Geometry: final body of the model. Coordinates: model frame, mm. A direction names the side the tool comes from. Give positions to 0.01 mm unless a question says otherwise; leave off trailing zeros. Write each loop counter-clockwise with the first axis right and the second up, starting at its lowest first coordinate (ties: lowest second). Pieces come first, ordered by that corner, then holes. Notation, with made-up numbers: (85.5, 85) -> (116.5, 85) arc R16 ccw to (116.5, 116) -> close; hole circle Ø9 at (66.5, 23). An arc over 180 degrees is marked (long way). Answer in a Markdown table with one row per item. Add a question column.
Item 1: First-contact query: P1, Ø4.5, axis at x = 12, z = -59.5, coming from the +Y side; P2, Ø2.5, axis at x = 48.94, z = -22.93, coming from the -Y side; P3, Ø4.5, axis at x = 12.065, z = -95.25, coming from the +Y side. Flat tips, straight axial feed; report the tip coordinate or a pass-through.
Item 2: Section query A-A on z = -53. Output: boundary loops of the cut face in (x, y) (3 decimals), plus the area to 3 significant figures.
Item 3: Material intervals for probe 1 along Z at (x, y) = (110, 11); probe 2 along Z at (x, y) = (61.5, 7); probe 3 along Z at (x, y) = (110.49, 6), sorted ascending. Write a range as from..to.
Item 4: Access query for faces 1 (the cylindrical face through (13.91, 5.01, -43.68)), 2 (the flat face through (108.06, 13.38, -10.78)), 3 (the flat face through (88.579, 3.131, -83.466)). Directions: +Z, -Z, +X, -X, +Y, -Y. A direction counts if a zero-diameter tool reaches every point of the face in a straight line with its end or side. Return the directions, or none.
Item 5: Section query C-C on y = 1.5. State how many separate pieces and enclosed holes the cut face has, plus the area to 3 significant figures.
Item 6: Section query B-B on x = 81.5. Output: boundary loops of the cut face in (y, z), plus the area to 3 significant figures.
Item 7: Draft query along X for faces 4 (the cylindrical face through (121.831, 8.371, -103.884)), 5 (the flat face through (86, 3, -19.765)). Return one class per face: +X half, -X half, draft (parallel to the pull), parting line (faces both ways), or undercut.
```python
from build123d import *

# Parameters (mm, degrees)
SKETCH2_W               = 122.555
SKETCH2_H               = 104.648
SKETCH2_R               = 2
SKETCH2_W_2             = 74.295
SKETCH2_H_2             = 69.53
BOSS_EXTRUDE5_DEPTH     = 16.51
SKETCH2_4_W             = 74.295
SKETCH2_4_H             = 10
SKETCH2_4_R             = 2
BOSS_EXTRUDE7_DEPTH     = 10.16
CUT_EXTRUDE1_START      = -16.51
SKETCH3_R               = 2
CUT_EXTRUDE1_DEPTH      = 6.35
FILLET1_R               = 2.54
CUT_EXTRUDE2_START      = -10.16
SKETCH4_R               = 2
CUT_EXTRUDE2_DEPTH      = 6.35
SKETCH5_R               = 2
CUT_EXTRUDE3_DEPTH      = 6.35
SKETCH6_R               = 2
CUT_EXTRUDE4_DEPTH      = 6.35
SKETCH7_R               = 2.254
SKETCH7_R_2             = 2
SUPPORTS_3D_PRINT_DEPTH = 6.35


with BuildPart() as part:
    # Sketch2 → Boss-Extrude5 (new body)
    with BuildSketch(Plane(origin=(0, 0, 0), x_dir=(1, 0, 0), z_dir=(0, 1, 0))):
        with Locations((61.2775, 52.324)):
            Rectangle(SKETCH2_W, SKETCH2_H)
        with Locations((12.065, 95.25)):
            Circle(SKETCH2_R, mode=Mode.SUBTRACT)
        with Locations((12.065, 60.198)):
            Circle(SKETCH2_R, mode=Mode.SUBTRACT)
        with Locations((12.065, 44.45)):
            Circle(SKETCH2_R, mode=Mode.SUBTRACT)
        with Locations((12.065, 9.398)):
            Circle(SKETCH2_R, mode=Mode.SUBTRACT)
        with Locations((110.49, 9.398)):
            Circle(SKETCH2_R, mode=Mode.SUBTRACT)
        with Locations((110.49, 44.45)):
            Circle(SKETCH2_R, mode=Mode.SUBTRACT)
        with Locations((110.49, 60.198)):
            Circle(SKETCH2_R, mode=Mode.SUBTRACT)
        with Locations((110.49, 95.25)):
            Circle(SKETCH2_R, mode=Mode.SUBTRACT)
        with Locations((73.744666667, 5.08)):
            Circle(SKETCH2_R, mode=Mode.SUBTRACT)
        with Locations((48.839129454, 5.150105129)):
            Circle(SKETCH2_R, mode=Mode.SUBTRACT)
        with Locations((61.2775, 52.324)):
            Rectangle(SKETCH2_W_2, SKETCH2_H_2, mode=Mode.SUBTRACT)
    extrude(amount=BOSS_EXTRUDE5_DEPTH)

    # Sketch2<4> → Boss-Extrude7 (add)
    with BuildSketch(Plane(origin=(0, 0, 0), x_dir=(1, 0, 0), z_dir=(0, 1, 0))):
        with Locations((61.2775, 22.559)):
            Rectangle(SKETCH2_4_W, SKETCH2_4_H)
        with Locations((36.533666667, 22.559)):
            Circle(SKETCH2_4_R, mode=Mode.SUBTRACT)
        with Locations((48.939224409, 22.929823378)):
            Circle(SKETCH2_4_R, mode=Mode.SUBTRACT)
        with Locations((61.341, 22.559)):
            Circle(SKETCH2_4_R, mode=Mode.SUBTRACT)
        with Locations((73.744666667, 22.86)):
            Circle(SKETCH2_4_R, mode=Mode.SUBTRACT)
        with Locations((86.148333333, 22.559)):
            Circle(SKETCH2_4_R, mode=Mode.SUBTRACT)
        with Locations((61.2775, 82.089)):
            Rectangle(SKETCH2_4_W, SKETCH2_4_H)
        with Locations((36.533666667, 82.089)):
            Circle(SKETCH2_4_R, mode=Mode.SUBTRACT)
        with Locations((61.341, 82.089)):
            Circle(SKETCH2_4_R, mode=Mode.SUBTRACT)
        with Locations((86.148333333, 82.089)):
            Circle(SKETCH2_4_R, mode=Mode.SUBTRACT)
    extrude(amount=BOSS_EXTRUDE7_DEPTH)

    # Sketch3 → Cut-Extrude1 (cut)
    with BuildSketch(Plane.XZ.offset(CUT_EXTRUDE1_START)):
        Polygon((13.678116652, -6.604), (10.451883348, -6.604), (8.838766696, -9.398), (10.451883348, -12.192), (13.678116652, -12.192), (15.291233304, -9.398), align=None)
        with Locations((12.065, -9.398)):
            Circle(SKETCH3_R, mode=Mode.SUBTRACT)
        Polygon((13.678116652, -92.456), (10.451883348, -92.456), (8.838766696, -95.25), (10.451883348, -98.044), (13.678116652, -98.044), (15.291233304, -95.25), align=None)
        with Locations((12.065, -95.25)):
            Circle(SKETCH3_R, mode=Mode.SUBTRACT)
        Polygon((112.103116652, -92.456), (108.876883348, -92.456), (107.263766696, -95.25), (108.876883348, -98.044), (112.103116652, -98.044), (113.716233304, -95.25), align=None)
        with Locations((110.49, -95.25)):
            Circle(SKETCH3_R, mode=Mode.SUBTRACT)
        Polygon((108.876883348, -12.192), (112.103116652, -12.192), (113.716233304, -9.398), (112.103116652, -6.604), (108.876883348, -6.604), (107.263766696, -9.398), align=None)
        with Locations((110.49, -9.398)):
            Circle(SKETCH3_R, mode=Mode.SUBTRACT)
        Polygon((13.678116652, -62.992), (15.291233304, -60.198), (13.678116652, -57.404), (10.451883348, -57.404), (8.838766696, -60.198), (10.451883348, -62.992), align=None)
        with Locations((12.065, -60.198)):
            Circle(SKETCH3_R, mode=Mode.SUBTRACT)
        Polygon((8.838766696, -44.45), (10.451883348, -47.244), (13.678116652, -47.244), (15.291233304, -44.45), (13.678116652, -41.656), (10.451883348, -41.656), align=None)
        with Locations((12.065, -44.45)):
            Circle(SKETCH3_R, mode=Mode.SUBTRACT)
        Polygon((107.263766696, -44.45), (108.876883348, -47.244), (112.103116652, -47.244), (113.716233304, -44.45), (112.103116652, -41.656), (108.876883348, -41.656), align=None)
        with Locations((110.49, -44.45)):
            Circle(SKETCH3_R, mode=Mode.SUBTRACT)
        Polygon((108.876883348, -57.404), (107.263766696, -60.198), (108.876883348, -62.992), (112.103116652, -62.992), (113.716233304, -60.198), (112.103116652, -57.404), align=None)
        with Locations((110.49, -60.198)):
            Circle(SKETCH3_R, mode=Mode.SUBTRACT)
    extrude(amount=CUT_EXTRUDE1_DEPTH, mode=Mode.SUBTRACT)

    # Fillet1
    fillet1_edges = [part.edges().sort_by_distance(p)[0] for p in [
        (0, 8.255, 0),
        (0, 8.255, -104.648),
        (122.555, 8.255, -104.648),
        (122.555, 8.255, 0),
    ]]
    fillet(fillet1_edges, radius=FILLET1_R)

    # Sketch4 → Cut-Extrude2 (cut)
    with BuildSketch(Plane(origin=(0, 10.16, 0), x_dir=(1, 0, 0), z_dir=(0, 1, 0)).offset(CUT_EXTRUDE2_START)):
        Polygon((39.759899971, 22.559), (38.146783319, 25.353), (34.920550015, 25.353), (33.307433362, 22.559), (34.920550015, 19.765), (38.146783319, 19.765), align=None)
        with Locations((36.533666667, 22.559)):
            Circle(SKETCH4_R, mode=Mode.SUBTRACT)
        Polygon((58.114766696, 22.559), (59.727883348, 19.765), (62.954116652, 19.765), (64.567233304, 22.559), (62.954116652, 25.353), (59.727883348, 25.353), align=None)
        with Locations((61.341, 22.559)):
            Circle(SKETCH4_R, mode=Mode.SUBTRACT)
        Polygon((82.922100029, 22.559), (84.535216681, 19.765), (87.761449985, 19.765), (89.374566638, 22.559), (87.761449985, 25.353), (84.535216681, 25.353), align=None)
        with Locations((86.148333333, 22.559)):
            Circle(SKETCH4_R, mode=Mode.SUBTRACT)
        Polygon((82.922100029, 82.089), (84.535216681, 79.295), (87.761449985, 79.295), (89.374566638, 82.089), (87.761449985, 84.883), (84.535216681, 84.883), align=None)
        with Locations((86.148333333, 82.089)):
            Circle(SKETCH4_R, mode=Mode.SUBTRACT)
        Polygon((64.567233304, 82.089), (62.954116652, 84.883), (59.727883348, 84.883), (58.114766696, 82.089), (59.727883348, 79.295), (62.954116652, 79.295), align=None)
        with Locations((61.341, 82.089)):
            Circle(SKETCH4_R, mode=Mode.SUBTRACT)
        Polygon((39.759899971, 82.089), (38.146783319, 84.883), (34.920550015, 84.883), (33.307433362, 82.089), (34.920550015, 79.295), (38.146783319, 79.295), align=None)
        with Locations((36.533666667, 82.089)):
            Circle(SKETCH4_R, mode=Mode.SUBTRACT)
    extrude(amount=CUT_EXTRUDE2_DEPTH, mode=Mode.SUBTRACT)

    # Sketch5 → Cut-Extrude3 (cut)
    with BuildSketch(Plane(origin=(0, 10.16, 0), x_dir=(1, 0, 0), z_dir=(0, 1, 0))):
        with Locations((48.839129454, 5.150105129)):
            Circle(SKETCH5_R)
        with Locations((73.744666667, 5.08)):
            Circle(SKETCH5_R)
        Polygon((76.970899971, 22.86), (75.357783319, 25.654), (72.131550015, 25.654), (70.518433362, 22.86), (72.131550015, 20.066), (75.357783319, 20.066), align=None)
        with Locations((73.744666667, 22.86)):
            Circle(SKETCH5_R, mode=Mode.SUBTRACT)
        Polygon((52.165457714, 22.929823378), (50.552341061, 25.723823378), (47.326107757, 25.723823378), (45.712991105, 22.929823378), (47.326107757, 20.135823378), (50.552341061, 20.135823378), align=None)
        with Locations((48.939224409, 22.929823378)):
            Circle(SKETCH5_R, mode=Mode.SUBTRACT)
    extrude(amount=-CUT_EXTRUDE3_DEPTH, mode=Mode.SUBTRACT)

    # Sketch6 → Cut-Extrude4 (cut)
    with BuildSketch(Plane(origin=(0, 16.51, 0), x_dir=(1, 0, 0), z_dir=(0, 1, 0))):
        Polygon((70.518433362, 5.08), (72.131550015, 2.286), (75.357783319, 2.286), (76.970899971, 5.08), (75.357783319, 7.874), (72.131550015, 7.874), align=None)
        with Locations((73.744666667, 5.08)):
            Circle(SKETCH6_R, mode=Mode.SUBTRACT)
        Polygon((45.612896149, 5.150105129), (47.226012801, 2.356105129), (50.452246106, 2.356105129), (52.065362758, 5.150105129), (50.452246106, 7.944105129), (47.226012801, 7.944105129), align=None)
        with Locations((48.839129454, 5.150105129)):
            Circle(SKETCH6_R, mode=Mode.SUBTRACT)
    extrude(amount=-CUT_EXTRUDE4_DEPTH, mode=Mode.SUBTRACT)

    # Sketch7 → Supports - 3D Print (add)
    with BuildSketch(Plane.XZ.offset(-6.35)):
        with Locations((36.533666667, -82.089)):
            Circle(SKETCH7_R)
        with Locations((36.533666667, -82.089)):
            Circle(SKETCH7_R_2, mode=Mode.SUBTRACT)
        with Locations((61.341, -82.089)):
            Circle(SKETCH7_R)
        with Locations((61.341, -82.089)):
            Circle(SKETCH7_R_2, mode=Mode.SUBTRACT)
        with Locations((86.148333333, -82.089)):
            Circle(SKETCH7_R)
        with Locations((86.148333333, -82.089)):
            Circle(SKETCH7_R_2, mode=Mode.SUBTRACT)
        with Locations((86.148333333, -22.559)):
            Circle(SKETCH7_R)
        with Locations((86.148333333, -22.559)):
            Circle(SKETCH7_R_2, mode=Mode.SUBTRACT)
        with Locations((61.341, -22.559)):
            Circle(SKETCH7_R)
        with Locations((61.341, -22.559)):
            Circle(SKETCH7_R_2, mode=Mode.SUBTRACT)
        with Locations((36.533666667, -22.559)):
            Circle(SKETCH7_R)
        with Locations((36.533666667, -22.559)):
            Circle(SKETCH7_R_2, mode=Mode.SUBTRACT)
    extrude(amount=SUPPORTS_3D_PRINT_DEPTH)


solid = part.part
```
Findings below:
| question | item | result |
|---|---|---|
| 1 | P1 | stops at y = 16.51 |
| 1 | P2 | passes through |
| 1 | P3 | stops at y = 10.16 |
| 2 | outline | (0, 0) -> (24.13, 0) -> (24.13, 16.51) -> (0, 16.51) -> close; (98.425, 0) -> (122.555, 0) -> (122.555, 16.51) -> (98.425, 16.51) -> close |
| 2 | area | 797 mm^2 |
| 3 | probe 1 | z = -104.65..-98.04, -92.46..-62.99, -57.4..-47.24, -41.66..-12.19, -6.6..0 |
| 3 | probe 2 | z = -104.65..-84.08, -80.1..-77.09, -27.56..-24.55, -20.57..0 |
| 3 | probe 3 | z = -104.65..-97.25, -93.25..-62.2, -58.2..-46.45, -42.45..-11.4, -7.4..0 |
| 4 | face 1 | +Y, -Y |
| 4 | face 2 | +Y |
| 4 | face 3 | -Y |
| 5 | separate pieces | 7 |
| 5 | enclosed holes | 25 |
| 5 | area | 8,850 mm^2 |
| 6 | outline | (0, -104.65) -> (16.51, -104.65) -> (16.51, -87.09) -> (10.16, -87.09) -> (10.16, -77.09) -> (0, -77.09) -> close; (0, -27.56) -> (10.16, -27.56) -> (10.16, -17.56) -> (16.51, -17.56) -> (16.51, 0) -> (0, 0) -> close |
| 6 | area | 783 mm^2 |
| 7 | face 4 | +X half |
| 7 | face 5 | undercut |
